Model file for the job. Use its own axes, mm. A direction names the side the tool comes from. Round coordinates to 2 decimals unless told otherwise and drop trailing zeros. Loops run counter-clockwise (first coordinate to the right, second up) from the corner with the lowest first, then second, coordinate; pieces in that order, holes last. Notation, with made-up numbers: M 70,56.5 L 91,56.5 A5 ccw 91,62.5 Z; hole C -10,74 d6. An arc over 180 degrees is marked long. Answer in a Markdown table with one row per item.
from build123d import *

# Parameters (mm, degrees)
ESBO_O1_W                = 26
ESBO_O1_H                = 19
RESSALTO_EXTRUS_O1_DEPTH = 1.6
ESBO_O2_W                = 1
ESBO_O2_H                = 2
RESSALTO_EXTRUS_O2_DEPTH = 0.5
ESBO_O3_W                = 9
ESBO_O3_H                = 7.4
RESSALTO_EXTRUS_O3_DEPTH = 3.2
FILETE1_R                = 1
FILETE7_R                = 1
CORTE_EXTRUS_O1_DEPTH    = 5.2
RESSALTO_EXTRUS_O4_REACH = 22.2
ESBO_O5_W                = 6
ESBO_O5_H                = 0.5
ESBO_O6_W                = 6.7
ESBO_O6_H                = 7.8
RESSALTO_EXTRUS_O5_DEPTH = 2.8
FILETE8_R                = 0.5
ESBO_O7_W                = 2.3
ESBO_O7_H                = 4.5
RESSALTO_EXTRUS_O6_DEPTH = 1.9
ESBO_O8_W                = 0.8
ESBO_O8_H                = 2
RESSALTO_EXTRUS_O7_DEPTH = 0.9
RESSALTO_EXTRUS_O7_TAPER = 2
ESBO_O9_W                = 13.1
ESBO_O9_H                = 13.7
RESSALTO_EXTRUS_O8_DEPTH = 8
ESBO_O10_W               = 13.1
ESBO_O10_H               = 1.3
CORTE_EXTRUS_O2_DEPTH    = 9
ESBO_O11_W               = 11.1
ESBO_O11_H               = 4.7
CORTE_EXTRUS_O3_DEPTH    = 9
RESSALTO_EXTRUS_O9_REACH = 22.2
ESBO_O12_W               = 10.5
ESBO_O12_H               = 2
CHANFRO1_SIZE            = 1
CHANFRO1_SIZE2           = 0.176326981
CHANFRO1_PART_2_SIZE     = 1
CHANFRO1_PART_2_SIZE2    = 0.176326981
CHANFRO1_PART_3_SIZE     = 1
CHANFRO1_PART_3_SIZE2    = 0.176326981
CHANFRO1_PART_4_SIZE     = 1
CHANFRO1_PART_4_SIZE2    = 0.176326981
CORTE_EXTRUS_O4_REACH    = 11.6
ESBO_O13_R               = 1


with BuildPart() as part:
    # Esboço1 → Ressalto-extrusão1 (new body)
    with BuildSketch(Plane.XY):
        with Locations((-18.344966746, 5.985294118)):
            Rectangle(ESBO_O1_W, ESBO_O1_H)
    extrude(amount=RESSALTO_EXTRUS_O1_DEPTH)

    # Esboço2 → Ressalto-extrusão2 (add)
    with BuildSketch(Plane.XY.offset(1.6)):
        with Locations((-27.844966746, 13.985294118)):
            Rectangle(ESBO_O2_W, ESBO_O2_H)
        with Locations((-25.844966746, 13.985294118)):
            Rectangle(ESBO_O2_W, ESBO_O2_H)
        with Locations((-23.844966746, 13.985294118)):
            Rectangle(ESBO_O2_W, ESBO_O2_H)
        with Locations((-21.844966746, 13.985294118)):
            Rectangle(ESBO_O2_W, ESBO_O2_H)
    extrude(amount=RESSALTO_EXTRUS_O2_DEPTH)

    # Esboço3 → Ressalto-extrusão3 (add)
    with BuildSketch(Plane.XY.offset(1.6)):
        with Locations((-13.244966746, 12.985294118)):
            Rectangle(ESBO_O3_W, ESBO_O3_H)
    extrude(amount=RESSALTO_EXTRUS_O3_DEPTH)

    # Filete1
    filete1_edges = [part.edges().sort_by_distance(p)[0] for p in [
        (-8.744966746, 12.985294118, 4.8),
    ]]
    fillet(filete1_edges, radius=FILETE1_R)

    # Filete7
    filete7_edges = [part.edges().sort_by_distance(p)[0] for p in [
        (-17.744966746, 16.085294118, 1.6),
        (-8.744966746, 16.085294118, 1.6),
        (-17.744966746, 12.985294118, 4.8),
    ]]
    fillet(filete7_edges, radius=FILETE7_R)

    # Esboço4 → Corte-extrusão1 (cut)
    with BuildSketch(Plane(origin=(0, 16.685294118, 0), x_dir=(1, 0, 0), z_dir=(0, 1, 0))):
        with BuildLine():
            Line((-9.744966746, -1.9), (-16.744966746, -1.9))
            ThreePointArc((-16.744966746, -1.9), (-17.239941493, -2.105025253), (-17.444966746, -2.6))
            Line((-17.444966746, -2.6), (-17.444966746, -3.8))
            ThreePointArc((-17.444966746, -3.8), (-17.239941493, -4.294974747), (-16.744966746, -4.5))
            Line((-16.744966746, -4.5), (-9.744966746, -4.5))
            ThreePointArc((-9.744966746, -4.5), (-9.249991999, -4.294974747), (-9.044966746, -3.8))
            Line((-9.044966746, -3.8), (-9.044966746, -2.6))
            ThreePointArc((-9.044966746, -2.6), (-9.249991999, -2.105025253), (-9.744966746, -1.9))
        make_face()
    extrude(amount=-CORTE_EXTRUS_O1_DEPTH, mode=Mode.SUBTRACT)

    # Esboço5 → Ressalto-extrusão4 (add, up to next)
    with BuildSketch(Plane(origin=(0, 16.685294118, 0), x_dir=(1, 0, 0), z_dir=(0, 1, 0)), mode=Mode.PRIVATE) as ressalto_extrus_o4_sk1:
        with Locations((-13.539619271, -3.2)):
            Rectangle(ESBO_O5_W, ESBO_O5_H)
    ressalto_extrus_o4_tool1 = extrude(ressalto_extrus_o4_sk1.sketch, amount=-RESSALTO_EXTRUS_O4_REACH, mode=Mode.PRIVATE) - part.part
    add(ressalto_extrus_o4_tool1.solids().sort_by_distance((-13.539619, 16.685294, 3.2))[0])

    # Esboço6 → Ressalto-extrusão5 (add)
    with BuildSketch(Plane.XY.offset(1.6)):
        with Locations((-12.494966746, 3.885294118)):
            Rectangle(ESBO_O6_W, ESBO_O6_H)
    extrude(amount=RESSALTO_EXTRUS_O5_DEPTH)

    # Filete8
    filete8_edges = [part.edges().sort_by_distance(p)[0] for p in [
        (-15.844966746, 7.785294118, 3),
        (-15.844966746, -0.014705882, 3),
        (-9.144966746, -0.014705882, 3),
        (-9.144966746, 7.785294118, 3),
    ]]
    fillet(filete8_edges, radius=FILETE8_R)

    # Esboço7 → Ressalto-extrusão6 (add)
    with BuildSketch(Plane.XY.offset(1.6)):
        with Locations((-29.994966746, 4.435294118)):
            Rectangle(ESBO_O7_W, ESBO_O7_H)
    extrude(amount=RESSALTO_EXTRUS_O6_DEPTH)

    # Esboço8 → Ressalto-extrusão7 (add)
    with BuildSketch(Plane.ZY.offset(31.144966746)):
        with Locations((2.55, 4.435294118)):
            Rectangle(ESBO_O8_W, ESBO_O8_H)
    extrude(amount=RESSALTO_EXTRUS_O7_DEPTH, taper=RESSALTO_EXTRUS_O7_TAPER)

    # Esboço9 → Ressalto-extrusão8 (add)
    with BuildSketch(Plane(origin=(0, 0, 0), x_dir=(-1, 0, 0), z_dir=(0, 0, -1))):
        with Locations((15.594966746, 9.835294118)):
            Rectangle(ESBO_O9_W, ESBO_O9_H)
    extrude(amount=RESSALTO_EXTRUS_O8_DEPTH)

    # Esboço10 → Corte-extrusão2 (cut)
    with BuildSketch(Plane(origin=(0, 16.685294118, 0), x_dir=(1, 0, 0), z_dir=(0, 1, 0))):
        with Locations((-15.594966746, 0.65)):
            Rectangle(ESBO_O10_W, ESBO_O10_H)
    extrude(amount=-CORTE_EXTRUS_O2_DEPTH, mode=Mode.SUBTRACT)

    # Esboço11 → Corte-extrusão3 (cut)
    with BuildSketch(Plane(origin=(0, 16.685294118, 0), x_dir=(1, 0, 0), z_dir=(0, 1, 0))):
        with Locations((-15.594966746, 4.65)):
            Rectangle(ESBO_O11_W, ESBO_O11_H)
    extrude(amount=-CORTE_EXTRUS_O3_DEPTH, mode=Mode.SUBTRACT)

    # Esboço12 → Ressalto-extrusão9 (add, up to next)
    with BuildSketch(Plane(origin=(0, 16.685294118, 0), x_dir=(1, 0, 0), z_dir=(0, 1, 0)), mode=Mode.PRIVATE) as ressalto_extrus_o9_sk1:
        with Locations((-15.594966746, 5.7)):
            Rectangle(ESBO_O12_W, ESBO_O12_H)
    ressalto_extrus_o9_tool1 = extrude(ressalto_extrus_o9_sk1.sketch, amount=-RESSALTO_EXTRUS_O9_REACH, mode=Mode.PRIVATE) - part.part
    add(ressalto_extrus_o9_tool1.solids().sort_by_distance((-15.594967, 16.685294, -5.7))[0])

    # Chanfro1
    chanfro1_edges = [part.edges().sort_by_distance(p)[0] for p in [
        (-20.844966746, 16.685294118, -5.7),
    ]]
    chanfro1_side = [part.faces().sort_by_distance(p)[0] for p in [
        (-20.844966746, 12.185294118, -5.7),
    ]]
    chamfer(chanfro1_edges, length=CHANFRO1_SIZE, length2=CHANFRO1_SIZE2, reference=chanfro1_side[0])

    # Chanfro1 part 2
    chanfro1_part_2_edges = [part.edges().sort_by_distance(p)[0] for p in [
        (-15.594966746, 16.685294118, -4.7),
    ]]
    chanfro1_part_2_side = [part.faces().sort_by_distance(p)[0] for p in [
        (-15.594966746, 12.185294118, -4.7),
    ]]
    chamfer(chanfro1_part_2_edges, length=CHANFRO1_PART_2_SIZE, length2=CHANFRO1_PART_2_SIZE2, reference=chanfro1_part_2_side[0])

    # Chanfro1 part 3
    chanfro1_part_3_edges = [part.edges().sort_by_distance(p)[0] for p in [
        (-10.344966746, 16.685294118, -5.7),
    ]]
    chanfro1_part_3_side = [part.faces().sort_by_distance(p)[0] for p in [
        (-10.344966746, 12.185294118, -5.7),
    ]]
    chamfer(chanfro1_part_3_edges, length=CHANFRO1_PART_3_SIZE, length2=CHANFRO1_PART_3_SIZE2, reference=chanfro1_part_3_side[0])

    # Chanfro1 part 4
    chanfro1_part_4_edges = [part.edges().sort_by_distance(p)[0] for p in [
        (-15.594966746, 16.685294118, -6.7),
    ]]
    chanfro1_part_4_side = [part.faces().sort_by_distance(p)[0] for p in [
        (-15.594966746, 12.185294118, -6.7),
    ]]
    chamfer(chanfro1_part_4_edges, length=CHANFRO1_PART_4_SIZE, length2=CHANFRO1_PART_4_SIZE2, reference=chanfro1_part_4_side[0])

    # Esboço13 → Corte-extrusão4 (cut, up to next)
    with BuildSketch(Plane.XY.offset(1.6), mode=Mode.PRIVATE) as corte_extrus_o4_sk1:
        with Locations((-31.344966746, 10.485294118)):
            Circle(ESBO_O13_R)
    corte_extrus_o4_tool1 = extrude(corte_extrus_o4_sk1.sketch, amount=-CORTE_EXTRUS_O4_REACH, mode=Mode.PRIVATE) & part.part
    add(corte_extrus_o4_tool1.solids().sort_by_distance((-31.344967, 10.485294, 1.6))[0], mode=Mode.SUBTRACT)
    # Esboço13 → Corte-extrusão4 (cut, up to next)
    with BuildSketch(Plane.XY.offset(1.6), mode=Mode.PRIVATE) as corte_extrus_o4_sk2:
        with Locations((-5.344966746, 10.485294118)):
            Circle(ESBO_O13_R)
    corte_extrus_o4_tool2 = extrude(corte_extrus_o4_sk2.sketch, amount=-CORTE_EXTRUS_O4_REACH, mode=Mode.PRIVATE) & part.part
    add(corte_extrus_o4_tool2.solids().sort_by_distance((-5.344967, 10.485294, 1.6))[0], mode=Mode.SUBTRACT)


solid = part.part
1. Mould opens along X. For faces 6 (the cylindrical face through (-17.444, 13.037, 4.515)), 7 (the flat face through (-26, 14, 2.1)), 8 (the flat face through (-19, 6, 1.6)) say: +X half, -X half, draft (parallel to the pull), parting line (faces both ways), or undercut.
Verdict:
| item | result |
|---|---|
| face 6 | -X half |
| face 7 | draft |
| face 8 | undercut |
2. Saw through at A-A (y = 14.5). State how many separate pieces and enclosed holes the cut face has, and give its area (3 significant figures).
Verdict:
| item | result |
|---|---|
| separate pieces | 4 |
| enclosed holes | 2 |
| area | 110 mm² |
3. Saw through at B-B (z = 1). Write the cut outline in (x, y).
Verdict:
| item | result |
|---|---|
| outline | M -31.34,-3.51 L -5.34,-3.51 L -5.34,9.49 A1 cw -5.34,11.49 L -5.34,15.49 L -31.34,15.49 L -31.34,11.49 A1 cw -31.34,9.49 Z |
4. Wall check: probe 1 along X at (y, z) = (11.5, -6.25); probe 2 along Z at (x, y) = (-12.25, 13); probe 3 along Y at (x, z) = (-13.75, 2.25). Give the ranges that are in metal, low to high.
Verdict:
| item | result |
|---|---|
| probe 1 | x = -22.14 to -21.14, -20.84 to -10.34, -10.04 to -9.04 |
| probe 2 | z = -8 to -7, -6.7 to -4.7, -2.3 to -1.3, 0 to 1.9, 2.95 to 3.45, 4.5 to 4.8 |
| probe 3 | y = -0.01 to 7.79, 9.29 to 11.49 |
5. Pin check, flat tips, straight feed: pin 1 (2.5 mm diameter, centred on y = 9, z = -3.5, fed in from -X); pin 2 (0.6 mm diameter, centred on y = 14.5, z = 2, fed in from +X); pin 3 (2 mm diameter, centred on x = -12.5, z = -2, fed in from -Y). Stop position of each tip, or through.
Verdict:
| item | result |
|---|---|
| pin 1 | stops at x = -22.14 |
| pin 2 | stops at x = -8.74 |
| pin 3 | stops at y = 2.99 |
6. Saw through at D-D (z = -4.25). Write the cut outline in (x, y).
Verdict:
| item | result |
|---|---|
| outline | M -22.14,2.99 L -9.04,2.99 L -9.04,16.69 L -10.04,16.69 L -10.04,7.69 L -21.14,7.69 L -21.14,16.69 L -22.14,16.69 Z |
7. Tool access for faces 1 (the flat face through (-13, 16, 1.6)), 2 (the flat face through (-14, 14, 3.45)), 3 (the flat face through (-15.845, 4, 3)), 4 (the flat face through (-13, -0.015, 3)), 5 (the flat face through (-30, 4, 3.5)): list every direction of +Z, -Z, +X, -X, +Y, -Y with a clear straight run to the whole face (end or side of a thin tool).
Verdict:
| item | result |
|---|---|
| face 1 | +X, -X, +Y |
| face 2 | +Y |
| face 3 | +Z, -Y |
| face 4 | +Z, +X, -X, -Y |
| face 5 | +Z, -X, +Y, -Y |
8. Saw through at C-C (x = -25). Write the cut outline in (y, z).
Verdict:
| item | result |
|---|---|
| outline | M -3.51,0 L 15.49,0 L 15.49,1.6 L -3.51,1.6 Z |
